```python
from build123d import *

# Parameters (mm, degrees)
SKETCH3_R                = 5
BOSS_EXTRUDE2_DEPTH      = 100
BOSS_EXTRUDE2_DEPTH_BACK = 100
CUT_EXTRUDE5_DEPTH       = 101
CUT_EXTRUDE5_DEPTH_BACK  = 101
CHAMFER1_SIZE            = 0.5


with BuildPart() as part:
    # Sketch3 → Boss-Extrude2 (new body, two sides)
    with BuildSketch(Plane.XY) as boss_extrude2_sk:
        Circle(SKETCH3_R)
    extrude(amount=BOSS_EXTRUDE2_DEPTH)
    extrude(boss_extrude2_sk.sketch, amount=-BOSS_EXTRUDE2_DEPTH_BACK)

    # Sketch10 → Cut-Extrude5 (cut, two sides)
    with BuildSketch(Plane.XY) as cut_extrude5_sk:
        with BuildLine():
            Line((-2.5, 4.330127019), (2.5, 4.330127019))
            ThreePointArc((2.5, 4.330127019), (0, 5), (-2.5, 4.330127019))
        make_face()
    extrude(amount=CUT_EXTRUDE5_DEPTH, mode=Mode.SUBTRACT)
    extrude(cut_extrude5_sk.sketch, amount=-CUT_EXTRUDE5_DEPTH_BACK, mode=Mode.SUBTRACT)

    # Chamfer1
    chamfer1_edges = [part.edges().sort_by_distance(p)[0] for p in [
        (0, -5, -100),
        (0, -5, 100),
    ]]
    chamfer(chamfer1_edges, length=CHAMFER1_SIZE)


solid = part.part
```
Verification items for the finished model (mm, model axes). Round coordinates to 2 decimals unless told otherwise and drop trailing zeros. Order: outer loops, then holes, each group sorted by start corner. A loop starts at its lowest first (then second) coordinate and runs counter-clockwise, first axis right, second up.
1) Depth check by flat-ended pin: pin 1 (3 mm diameter, centred on y = 2.5, z = 0, fed in from +X); pin 2 (1 mm diameter, centred on y = 2.5, z = -71, fed in from +X). Enter the tip coordinate at first touch or a pass-through.
Geometry says:
pin 1: stops at x = 4.9
pin 2: stops at x = 4.58
2) Cross-section at A-A, the plane z = -62. Record the cut outline in (x, y), plus the area to 3 significant figures.
Geometry says:
outline: (-2.5, 4.33) arc R5 ccw (long way) to (2.5, 4.33) - close
area: 76.3 mm2
3) Material ranges on line 1 (X direction, y = 0.25, z = -43); line 2 (X direction, y = -4, z = 16); line 3 (Y direction, x = 1, z = -14.5), recorded low to high.
Geometry says:
line 1: x = -4.99 to 4.99
line 2: x = -3 to 3
line 3: y = -4.9 to 4.33
